The model under review builds one solid part; all positions refer to its coordinate system, in mm. A direction names the side the tool comes from. Give positions to 0.01 mm unless a question says otherwise; leave off trailing zeros. Order: outer loops, then holes, each group sorted by start corner. A loop starts at its lowest first (then second) coordinate and runs counter-clockwise, first axis right, second up. Notation, with made-up numbers: (69, 19) -> (104, 19) arc R27 cw to (104, 58) -> close; hole circle Ø9 at (54, 42.25). An arc over 180 degrees is marked (long way). Use one line per item in the form item = value.
```python
from build123d import *

# Parameters (mm, degrees)
F6_DEPTH  = 1.2
F7_SIZE   = 0.99999
F11_DEPTH = 1.8


# Not quite as in the source:
# - a fillet or chamfer is up to 0.001 mm smaller than in the source, because OpenCascade refuses the exact size
# - a pattern or mirror of a feature is missing from the dataset's text; its kind, count and spacing are read off the source's solid


with BuildPart() as f1:
    # F0 (on Right) → F1 (revolve)
    with BuildSketch(Plane.YZ):
        Polygon((0, 4), (0, 0), (51, 0), (51, 4), (37.5, 4), (37.5, 5), (13.5, 5), (13.5, 4), align=None)
    revolve(axis=Axis((0, 25.5, 0), (0, -1, 0)))

    # F5 (on offset) → F6 (cut)
    with BuildSketch(Plane.XY.offset(4)):
        with BuildLine():
            Line((1, 8.5), (1, 11))
            ThreePointArc((1, 11), (0, 12), (-1, 11))
            Line((-1, 11), (-1, 8.5))
            ThreePointArc((-1, 8.5), (0, 7.5), (1, 8.5))
        make_face()
    f6 = extrude(amount=-F6_DEPTH, mode=Mode.SUBTRACT)

    # F6_copies: F6 across plane
    add(f6.mirror(Plane(origin=(-1e-06, 25.499997, -1e-06), x_dir=(0, 0, 1), z_dir=(0, 1, 0))), mode=Mode.SUBTRACT)

    # F7 (size 1 in the source; OpenCascade refuses exactly that, so slightly less here)
    f7_edges = [f1.edges().sort_by_distance(p)[0] for p in [
        (0, 13.5, -5),
        (0, 37.5, -5),
        (0, 51, -4),
        (0, 0, -4),
    ]]
    chamfer(f7_edges, length=F7_SIZE)

    # F10 (on offset) → F11 (cut)
    with BuildSketch(Plane.XY.offset(5)):
        with BuildLine():
            Line((1.5, 23), (1.5, 29.5))
            ThreePointArc((1.5, 29.5), (0, 31), (-1.5, 29.5))
            Line((-1.5, 29.5), (-1.5, 23))
            ThreePointArc((-1.5, 23), (0, 21.5), (1.5, 23))
        make_face()
    extrude(amount=-F11_DEPTH, mode=Mode.SUBTRACT)


solid = f1.part
```
1. For pin 1 Ø0.5 at (y, z) = (9.5, 3.5) entering from -X; pin 2 Ø1.5 at (y, z) = (39.5, -3.5) entering from +X; pin 3 Ø2 at (x, y) = (-3.5, 16) entering from +Z; pin 4 Ø3 at (x, z) = (-3.5, -1.5) entering from +Y, all flat-tipped, find the tip position at first contact; note any pin that passes through.
Values:
pin_1 = -2.33
pin_2 = 2.9
pin_3 = 4.33
pin_4 = 51
2. The part is to be moulded in two halves that separate along Y. For faces 1 (the face through (0, 0, 0)), 2 (the face through (0, 39, 3)), 3 (the face through (0, 51, 0)), say which applies: +Y half, -Y half, draft (parallel to the pull), parting line (faces both ways), or undercut.
Values:
face_1 = -Y half
face_2 = undercut
face_3 = +Y half
3. Add section C-C on y = 38. Give the boundary of the cut face in (x, z), then the cut area to 3 significant figures.
Values:
outline = circle Ø8 at (0, 0)
area = 50.3 mm^2
4. Tool access review of faces 4 (the face through (3.905, 43.663, -0.867)), 5 (the face through (4.88, 25.35, -1.08)), 6 (the face through (0, 41, 2.8)), 7 (the face through (3.905, 7.162, -0.867)): name each direction out of +Z, -Z, +X, -X, +Y, -Y from which nothing blocks a thin tool from reaching the whole face with its end or side.
Values:
face_4 = +Y
face_5 = +Y, -Y
face_6 = +Z
face_7 = -Y
5. Add section D-D on y = 32.5. Give the boundary of the cut face in (x, z), then the cut area to 3 significant figures.
Values:
outline = circle Ø10 at (0, 0)
area = 78.5 mm^2
6. For L1, parallel to X at y = 22, z = -3; L2, parallel to Z at x = -0.25, y = 2; L3, parallel to Y at x = -2, z = 4, list the stretches that pass through material, from the lowest coordinate up.
Values:
L1 = -4 to 4
L2 = -3.99 to 3.99
L3 = 13.97 to 37.03
